from build123d import *

# Parameters (mm, degrees)
F0_R     = 1.27
F1_DEPTH = 25.4
F2_W     = 1.0922
F2_H     = 3.81
F3_DEPTH = 9.398
F4_DEPTH = 25.4
F5_W     = 1.0922
F5_H     = 3.81
F6_DEPTH = 25.4
F7_DEPTH = 25.4
F8_DEPTH = 25.4


with BuildPart() as f1:
    # F0 (on Top) → F1 (new body)
    with BuildSketch(Plane.XY):
        Circle(F0_R)
    extrude(amount=F1_DEPTH)

    # F2 (on Front) → F3 (cut)
    with BuildSketch(Plane.XZ):
        with Locations((0, 26.14588)):
            Rectangle(F2_W, F2_H)
    extrude(amount=F3_DEPTH, mode=Mode.SUBTRACT)

    # F2 (on Front) → F4 (cut)
    with BuildSketch(Plane.XZ):
        with Locations((0, 26.14588)):
            Rectangle(F2_W, F2_H)
    extrude(amount=-F4_DEPTH, mode=Mode.SUBTRACT)

    # F5 (on Front) → F6 (cut)
    with BuildSketch(Plane.XZ):
        Rectangle(F5_W, F5_H)
    extrude(amount=-F6_DEPTH, mode=Mode.SUBTRACT)

    # F5 (on Front) → F7 (cut)
    with BuildSketch(Plane.XZ):
        Rectangle(F5_W, F5_H)
    extrude(amount=F7_DEPTH, mode=Mode.SUBTRACT)

    # F2 (on Front) → F8 (cut)
    with BuildSketch(Plane.XZ):
        with Locations((0, 26.14588)):
            Rectangle(F2_W, F2_H)
    extrude(amount=-F8_DEPTH, mode=Mode.SUBTRACT)


solid = f1.part
Verification items for the finished model (mm, model axes). A direction names the side the tool comes from. Round coordinates to 2 decimals unless told otherwise and drop trailing zeros. Write each loop counter-clockwise with the first axis right and the second up, starting at its lowest first coordinate (ties: lowest second). Pieces come first, ordered by that corner, then holes.
(1) Material ranges on line 1 (X direction, y = 0.1, z = 7.25); line 2 (Z direction, x = 0.25, y = -0.4) (3 decimals), recorded low to high.
Returned:
line 1: x = -1.27 to 1.27
line 2: z = 1.905 to 24.241
(2) Section check A-A (y = 0). Enter the section's corners in (x, z) (3 decimals), plus the area to 3 significant figures.
Returned:
outline: (-1.27, 0) - (-0.546, 0) - (-0.546, 1.905) - (0.546, 1.905) - (0.546, 0) - (1.27, 0) - (1.27, 25.4) - (0.546, 25.4) - (0.546, 24.241) - (-0.546, 24.241) - (-0.546, 25.4) - (-1.27, 25.4) - close
area: 61.2 mm2
(3) Mould release check, pull along X, two halves, no side actions. Record for faces 3 (the flat face through (-0.546, 0, 1)), 4 (the cylindrical face through (1.21, 0.38, 12.52)): pulls with the +X half, pulls with the -X half, needs draft (parallel to the pull), parting line crosses it, or undercut.
Returned:
face 3: undercut
face 4: parting line crosses it
(4) Access from +Z, -Z, +X, -X, +Y, -Y to the whole of each face (thin tool, end or side, straight path). Record for faces 1 (the flat face through (0.546, 0, 25)), 2 (the flat face through (0.546, 0, 1)).
Returned:
face 1: +Z, +Y, -Y
face 2: -Z, +Y, -Y
(5) Depth check by flat-ended pin: pin 1 Ø1.5 at (y, z) = (-1, 13.5) entering from +X; pin 2 Ø1.5 at (x, z) = (-1, 6.5) entering from +Y; pin 3 Ø0.9 at (x, y) = (0, -0.5) entering from +Z. Enter the tip coordinate at first touch or a pass-through.
Returned:
pin 1: stops at x = 1.25
pin 2: stops at y = 1.25
pin 3: stops at z = 24.24
(6) Section check B-B (x = 0). Enter the section's corners in (y, z) (3 decimals).
Returned:
outline: (-1.27, 1.905) - (1.27, 1.905) - (1.27, 24.241) - (-1.27, 24.241) - close
(7) Section check C-C (z = 3). Enter the section's corners in (x, y).
Returned:
outline: circle Ø2.54 at (0, 0)
